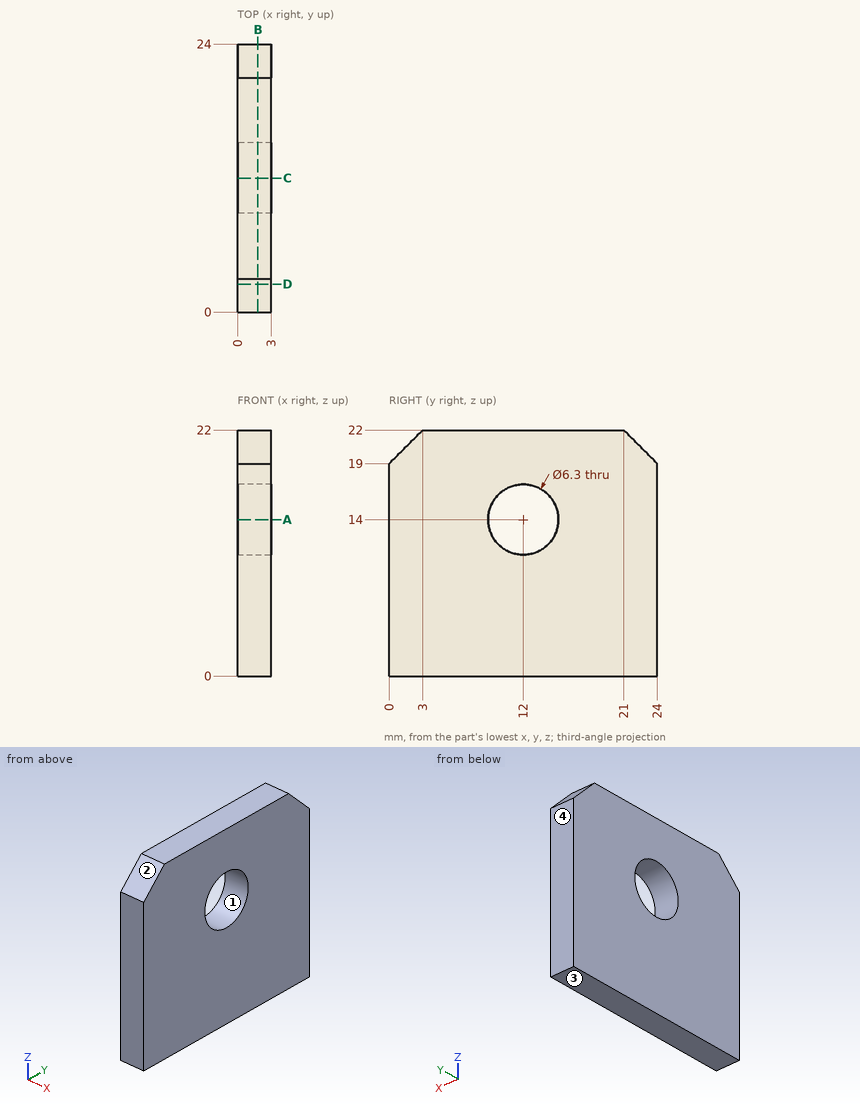
Verification items for this drawing (mm, ordinates from the low corner). Round coordinates to 2 decimals unless told otherwise and drop trailing zeros. Order: outer loops, then holes, each group sorted by start corner. A loop starts at its lowest first (then second) coordinate and runs counter-clockwise, first axis right, second up. Notation, with made-up numbers: (51.25, 70) - (91.25, 70) arc R17 cw to (91.25, 86) - close; hole circle Ø6 at (44, 69.25). An arc over 180 degrees is marked (long way). Answer as CSV lines item,"result". Start each with the question number.
1) Depth check by flat-ended pin: pin 1 (5 mm diameter, centred on y = 12, z = 14, fed in from -X). Enter the tip coordinate at first touch or a pass-through.
2) Section check B-B (x = 1.8). Record the cut outline in (y, z).
3) Scan lines: probe 1 along Z at (x, y) = (1.7, 12); probe 2 along Y at (x, z) = (0.9, 14); probe 3 along Y at (x, z) = (1.45, 16.5). Record each from-to range of solid material in increasing order.
4) Draft check along Y on the marked faces 1, 2, 3 and 4. Enter one of: +Y half, -Y half, draft (parallel to the pull), parting line (faces both ways), or undercut.
5) Section check D-D (y = 2.5). Record the cut outline in (x, z).
6) Section check C-C (y = 12). Record the cut outline in (x, z).
7) Section check A-A (z = 14). Record the cut outline in (x, y).
Determined:
1,pin 1,"through"
2,outline,"(0, 0) - (24, 0) - (24, 19) - (21, 22) - (3, 22) - (0, 19) - close; hole circle Ø6.3 at (12, 14)"
3,probe 1,"0 to 10.85, 17.15 to 22"
3,probe 2,"0 to 8.85, 15.15 to 24"
3,probe 3,"0 to 10.08, 13.92 to 24"
4,face 1,"undercut"
4,face 2,"-Y half"
4,face 3,"draft"
4,face 4,"+Y half"
5,outline,"(0, 0) - (3, 0) - (3, 21.5) - (0, 21.5) - close"
6,outline,"(0, 0) - (3, 0) - (3, 10.85) - (0, 10.85) - close; (0, 17.15) - (3, 17.15) - (3, 22) - (0, 22) - close"
7,outline,"(0, 0) - (3, 0) - (3, 8.85) - (0, 8.85) - close; (0, 15.15) - (3, 15.15) - (3, 24) - (0, 24) - close"
